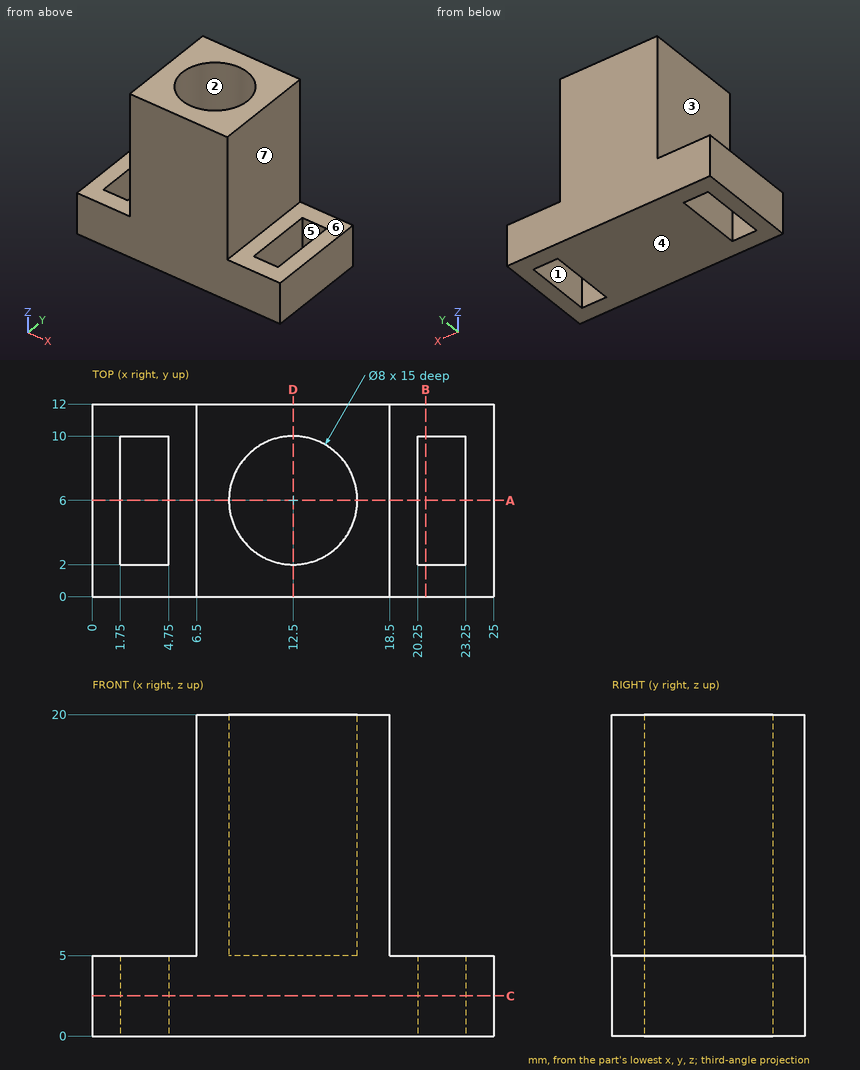
Geometry check sheet. Reference: drawing and pictorial views, mm from the part's lowest x, y, z. A direction names the side the tool comes from. Give positions to 0.01 mm unless a question says otherwise; leave off trailing zeros. Order: outer loops, then holes, each group sorted by start corner. A loop starts at its lowest first (then second) coordinate and runs counter-clockwise, first axis right, second up. Notation, with made-up numbers: M 1,39.5 L 44,39.5 A10 ccw 44,56.5 Z; hole C 79.5,9 d11. An arc over 180 degrees is marked long. Answer in a Markdown table with one row per item. Add a question column.
Q1. Gauge pin test, flat ends, axial feed: pin 1 Ø4 at (y, z) = (3.5, 14) entering from +X; pin 2 Ø1.5 at (y, z) = (8, 12) entering from -X; pin 3 Ø4 at (x, y) = (11, 6) entering from +Z. Record the tip position at first contact, or that the pin passes through.
Q2. Sectioned sample at D-D, the plane x = 12.5. Record the boundary of the cut face in (y, z), and give its area (3 significant figures).
Q3. Sectioned sample at C-C, the plane z = 2.5. Record the boundary of the cut face in (x, y), and give its area (3 significant figures).
Q4. Sectioned sample at B-B, the plane x = 20.75. Record the boundary of the cut face in (y, z), and give its area (3 significant figures).
Q5. Access from +Z, -Z, +X, -X, +Y, -Y to the whole of each face (thin tool, end or side, straight path). Record for the marked faces 1, 2, 3 and 4.
Q6. Sectioned sample at A-A, the plane y = 6. Record the boundary of the cut face in (x, z), and give its area (3 significant figures).
Q7. Thickness scan on L1, parallel to Y at x = 12.5, z = 16.25; L2, parallel to X at y = 4.5, z = 4.5; L3, parallel to Z at x = 12.5, y = 8.25. Record the ranges inside material, lowest first.
Q8. Release check for a two-part mould opening along X. For the marked faces 5, 6 and 7 record: released by +X, released by -X, zero draft, split by the parting line, or undercut.
Verdict:
| question | item | result |
|---|---|---|
| 1 | pin 1 | x = 18.5 |
| 1 | pin 2 | x = 6.5 |
| 1 | pin 3 | z = 5 |
| 2 | outline | M 0,0 L 12,0 L 12,20 L 10,20 L 10,5 L 2,5 L 2,20 L 0,20 Z |
| 2 | area | 120 mm² |
| 3 | outline | M 0,0 L 25,0 L 25,12 L 0,12 Z; hole M 1.75,2 L 4.75,2 L 4.75,10 L 1.75,10 Z; hole M 20.25,2 L 23.25,2 L 23.25,10 L 20.25,10 Z |
| 3 | area | 252 mm² |
| 4 | outline | M 0,0 L 2,0 L 2,5 L 0,5 Z; M 10,0 L 12,0 L 12,5 L 10,5 Z |
| 4 | area | 20.0 mm² |
| 5 | face 1 | +Z, -Z |
| 5 | face 2 | +Z |
| 5 | face 3 | +Z, -X, +Y, -Y |
| 5 | face 4 | -Z, +X, -X, +Y, -Y |
| 6 | outline | M 0,0 L 1.75,0 L 1.75,5 L 0,5 Z; M 4.75,0 L 20.25,0 L 20.25,5 L 18.5,5 L 18.5,20 L 16.5,20 L 16.5,5 L 8.5,5 L 8.5,20 L 6.5,20 L 6.5,5 L 4.75,5 Z; M 23.25,0 L 25,0 L 25,5 L 23.25,5 Z |
| 6 | area | 155 mm² |
| 7 | L1 | 0 to 2, 10 to 12 |
| 7 | L2 | 0 to 1.75, 4.75 to 20.25, 23.25 to 25 |
| 7 | L3 | 0 to 5 |
| 8 | face 5 | undercut |
| 8 | face 6 | zero draft |
| 8 | face 7 | released by +X |
